Can you work these out from the model? Positions are in its coordinate system, mm. Face numbers are marked on the shaded views. A direction names the side the tool comes from. Give positions to 0.01 mm unless a question says otherwise; leave off trailing zeros. Loops run counter-clockwise (first coordinate to the right, second up) from the corner with the lowest first, then second, coordinate; pieces in that order, holes last. Notation, with made-up numbers: (43.5, 49.25) - (62.5, 49.25) arc R15 ccw to (62.5, 61.25) - close; hole circle Ø11 at (14.25, -0.75). An arc over 180 degrees is marked (long way). Answer as a JSON object with one key per item and string values.
```python
from build123d import *

# Parameters (mm, degrees)
SKETCH1_W                   = 114.3
SKETCH1_H                   = 127
BOSS_EXTRUDE1_DEPTH         = 6.35
SKETCH2_W                   = 9.398
SKETCH2_H                   = 101.6
BOSS_EXTRUDE2_DEPTH         = 29.21
SKETCH10_R                  = 3.175
CUT_EXTRUDE1_DEPTH          = 115.596583549
SKETCH13_W                  = 2.667
SKETCH13_H                  = 6.35
CUT_EXTRUDE2_DEPTH          = 9.398
CUT_EXTRUDE3_REACH          = 92.286
SKETCH15_W                  = 25.4
SKETCH15_H                  = 25.4
MIRROR4_COPY_1_SKETCH_W     = 2.667
MIRROR4_COPY_1_SKETCH_H     = 6.35
MIRROR4_COPY_1_DEPTH        = 9.398
SKETCH19_W                  = 1.524
SKETCH19_H                  = 43.18
CUT_EXTRUDE4_DEPTH          = 5.08
SKETCH23_W                  = 5.842
SKETCH23_H                  = 11.43
CUT_EXTRUDE5_DEPTH          = 20.828
SKETCH24_W                  = 127.881325932
SKETCH24_H                  = 16.190143287
CUT_EXTRUDE6_DEPTH          = 12.7
SKETCH26_W                  = 20.33012471
SKETCH26_H                  = 111.91731712
CUT_EXTRUDE8_DEPTH          = 25.781
CHAMFER1_SIZE               = 3.81
SKETCH28_W                  = 17.78
SKETCH28_H                  = 12.7
BOSS_EXTRUDE3_DEPTH         = 12.7
SKETCH30_W                  = 11.43
SKETCH30_H                  = 5.842
CUT_EXTRUDE9_DEPTH          = 75.423408732
F_1_4_CLEARANCE_HOLE1_D     = 7.14248
F_1_4_CLEARANCE_HOLE1_DEPTH = 3.636839777
CHAMFER3_SIZE2              = 6.35
CHAMFER3_SIZE               = 2.54
F_1_4_CLEARANCE_HOLE2_D     = 7.14248
F_1_4_CLEARANCE_HOLE2_DEPTH = 15.24


with BuildPart() as part:
    # Sketch1 → Boss-Extrude1 (new body)
    with BuildSketch(Plane.XY):
        Rectangle(SKETCH1_W, SKETCH1_H)
    extrude(amount=BOSS_EXTRUDE1_DEPTH)

    # Sketch2 → Boss-Extrude2 (add)
    with BuildSketch(Plane.XY.offset(6.35)):
        with Locations((26.67, 0)):
            Rectangle(SKETCH2_W, SKETCH2_H)
    boss_extrude2 = extrude(amount=BOSS_EXTRUDE2_DEPTH)

    # Mirror1: Boss-Extrude2 across plane
    add(boss_extrude2.mirror(Plane(origin=(0, 0, 0), x_dir=(0, 0, 1), z_dir=(1, 0, 0))))

    # Sketch10 → Cut-Extrude1 (cut, through all)
    with BuildSketch(Plane(origin=(31.369, 0, 0), x_dir=(0, 0, -1), z_dir=(1, 0, 0))):
        with Locations((-22.86, 43.18)):
            Circle(SKETCH10_R)
    cut_extrude1 = extrude(amount=-CUT_EXTRUDE1_DEPTH, mode=Mode.SUBTRACT)

    # Mirror2: Cut-Extrude1 across plane
    add(cut_extrude1.mirror(Plane.ZX), mode=Mode.SUBTRACT)

    # Sketch13 → Cut-Extrude2 (cut)
    with BuildSketch(Plane(origin=(31.369, 0, 0), x_dir=(0, 0, -1), z_dir=(1, 0, 0))):
        with Locations((-30.5435, 43.18)):
            Rectangle(SKETCH13_W, SKETCH13_H)
    cut_extrude2 = extrude(amount=-CUT_EXTRUDE2_DEPTH, mode=Mode.SUBTRACT)

    # Sketch15 → Cut-Extrude3 (cut, up to next)
    with BuildSketch(Plane.XY.offset(6.35), mode=Mode.PRIVATE) as cut_extrude3_sk1:
        with Locations((-5.08, 0)):
            Rectangle(SKETCH15_W, SKETCH15_H)
    cut_extrude3_tool1 = extrude(cut_extrude3_sk1.sketch, amount=-CUT_EXTRUDE3_REACH, mode=Mode.PRIVATE) & part.part
    add(cut_extrude3_tool1.solids().sort_by_distance((-5.08, 0, 6.35))[0], mode=Mode.SUBTRACT)

    # Sketch16 → #4 Clearance Hole1 (revolve, cut)
    with BuildSketch(Plane(origin=(26.67, 43.18, 35.56), x_dir=(0, -1, 0), z_dir=(1, 0, 0))):
        Polygon((0, 0), (0, 12.918574487), (1.63195, 11.938), (1.63195, 0), align=None)
    f_4_clearance_hole1 = revolve(axis=Axis((26.67, 43.18, 41.91), (0, 0, -1)), mode=Mode.SUBTRACT)

    # Mirror3: Cut-Extrude2, #4 Clearance Hole1 across plane
    add(cut_extrude2.mirror(Plane(origin=(0, 0, 0), x_dir=(0, 0, 1), z_dir=(1, 0, 0))), mode=Mode.SUBTRACT)
    add(f_4_clearance_hole1.mirror(Plane(origin=(0, 0, 0), x_dir=(0, 0, 1), z_dir=(1, 0, 0))), mode=Mode.SUBTRACT)

    # Mirror4: Cut-Extrude2, #4 Clearance Hole1 across plane
    add(cut_extrude2.mirror(Plane.ZX), mode=Mode.SUBTRACT)
    add(f_4_clearance_hole1.mirror(Plane.ZX), mode=Mode.SUBTRACT)

    # Mirror4 copy 1 sketch → Mirror4 copy 1 (cut)
    with BuildSketch(Plane(origin=(-31.369, 0, 0), x_dir=(0, 0, -1), z_dir=(-1, 0, 0))):
        with Locations((-30.5435, 43.18)):
            Rectangle(MIRROR4_COPY_1_SKETCH_W, MIRROR4_COPY_1_SKETCH_H)
    extrude(amount=-MIRROR4_COPY_1_DEPTH, mode=Mode.SUBTRACT)

    # Mirror4 copy 2 sketch → Mirror4 copy 2 (revolve, cut)
    with BuildSketch(Plane(origin=(-26.67, -43.18, 35.56), x_dir=(0, 1, 0), z_dir=(-1, 0, 0))):
        Polygon((0, 0), (0, 12.918574487), (1.63195, 11.938), (1.63195, 0), align=None)
    revolve(axis=Axis((-26.67, -43.18, 41.91), (0, 0, -1)), mode=Mode.SUBTRACT)

    # Sketch19 → Cut-Extrude4 (cut)
    with BuildSketch(Plane(origin=(-21.971, 0, 0), x_dir=(0, 0, -1), z_dir=(1, 0, 0))):
        with Locations((-22.86, 0)):
            Rectangle(SKETCH19_W, SKETCH19_H)
    extrude(amount=-CUT_EXTRUDE4_DEPTH, mode=Mode.SUBTRACT)

    # Sketch23 → Cut-Extrude5 (cut)
    with BuildSketch(Plane.XY.offset(35.56)):
        with Locations((26.67, 0)):
            Rectangle(SKETCH23_W, SKETCH23_H)
    extrude(amount=-CUT_EXTRUDE5_DEPTH, mode=Mode.SUBTRACT)

    # Sketch24 → Cut-Extrude6 (cut)
    with BuildSketch(Plane(origin=(0, 63.5, 0), x_dir=(1, 0, 0), z_dir=(0, 1, 0))):
        with Locations((0, -3.427395894)):
            Rectangle(SKETCH24_W, SKETCH24_H)
    cut_extrude6 = extrude(amount=-CUT_EXTRUDE6_DEPTH, mode=Mode.SUBTRACT)

    # Mirror5: Cut-Extrude6 across plane
    add(cut_extrude6.mirror(Plane.ZX), mode=Mode.SUBTRACT)

    # Sketch26 → Cut-Extrude8 (cut)
    with BuildSketch(Plane(origin=(57.15, 0, 0), x_dir=(0, 0, -1), z_dir=(1, 0, 0))):
        with Locations((-3.366450344, 0)):
            Rectangle(SKETCH26_W, SKETCH26_H)
    cut_extrude8 = extrude(amount=-CUT_EXTRUDE8_DEPTH, mode=Mode.SUBTRACT)

    # Mirror6: Cut-Extrude8 across plane
    add(cut_extrude8.mirror(Plane(origin=(0, 0, 0), x_dir=(0, 0, 1), z_dir=(1, 0, 0))), mode=Mode.SUBTRACT)

    # Chamfer1
    chamfer1_edges = [part.edges().sort_by_distance(p)[0] for p in [
        (0, 50.8, 0),
    ]]
    chamfer(chamfer1_edges, length=CHAMFER1_SIZE)

    # Sketch28 → Boss-Extrude3 (add)
    with BuildSketch(Plane.XZ.offset(50.8)):
        with Locations((0, 6.35)):
            Rectangle(SKETCH28_W, SKETCH28_H)
    extrude(amount=BOSS_EXTRUDE3_DEPTH)

    # Sketch30 → Cut-Extrude9 (cut, through all)
    with BuildSketch(Plane.XY.offset(12.7)):
        with Locations((0.067049503, -56.942160223)):
            Rectangle(SKETCH30_W, SKETCH30_H)
    extrude(amount=-CUT_EXTRUDE9_DEPTH, mode=Mode.SUBTRACT)

    # 1/4 Clearance Hole1
    with Locations(Plane(origin=(0, -63.5, 0), x_dir=(-1, 0, 0), z_dir=(0, -1, 0))):
        with Locations((0, -6.35)):
            Hole(F_1_4_CLEARANCE_HOLE1_D / 2, depth=F_1_4_CLEARANCE_HOLE1_DEPTH)

    # Chamfer3
    chamfer3_edges = [part.edges().sort_by_distance(p)[0] for p in [
        (0, -50.8, 12.7),
    ]]
    chamfer3_side = [part.faces().sort_by_distance(p)[0] for p in [
        (0, -50.8508, 12.7),
    ]]
    chamfer(chamfer3_edges, length=CHAMFER3_SIZE - 0.0001, length2=CHAMFER3_SIZE2 - 0.0001, reference=chamfer3_side[0])  # a hair under: the kernel refuses the full size

    # 1/4 Clearance Hole2
    with Locations(Plane(origin=(31.369, 0, 0), x_dir=(0, 0, -1), z_dir=(1, 0, 0))):
        with Locations((-21.082, 0)):
            Hole(F_1_4_CLEARANCE_HOLE2_D / 2, depth=F_1_4_CLEARANCE_HOLE2_DEPTH)


solid = part.part
```
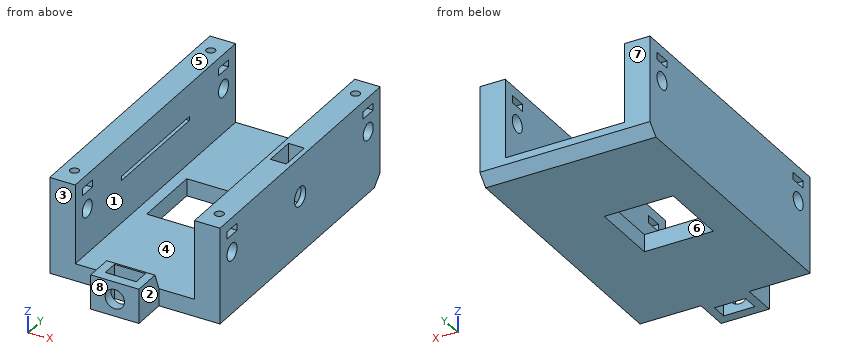
1) I'm going to push flat-ended pins straight in: P1, Ø1.3, axis at x = 28.5, z = 30.5, coming from the -Y side; P2, Ø12, axis at x = 2.5, y = 26.5, coming from the +Z side; P3, Ø14, axis at y = -59, z = 6, coming from the -X side. Where does each tip first touch, or does it pass through?
Check sheet entries:
{"P1": "y = -50.8", "P2": "z = 6.35", "P3": "x = -8.89"}
2) I need wall thicknesses on L1, parallel to X at y = 43, z = 34; L2, parallel to Y at x = -26.67, z = 27.45; L3, parallel to X at y = -36, z = 27.5. Which ranges of each line are inside material? Lowest first, please.
Check sheet entries:
{"L1": "-31.37 to -28.29, -25.05 to -21.97, 21.97 to 25.05, 28.29 to 31.37", "L2": "-50.8 to -44.81, -41.55 to 41.55, 44.81 to 50.8", "L3": "-31.37 to -21.97, 21.97 to 31.37"}
3) Imagine slicing it at C-C on y = -26.5. Write out the boundary of the cut face in (x, z).
Check sheet entries:
{"outline": "(-31.37, 0) - (31.37, 0) - (31.37, 35.56) - (21.97, 35.56) - (21.97, 6.35) - (-21.97, 6.35) - (-21.97, 35.56) - (-31.37, 35.56) - close"}
4) Imagine slicing it at A-A on x = -15. Write out the boundary of the cut face in (y, z), and give its area (3 significant figures).
Check sheet entries:
{"outline": "(-50.8, 0) - (-12.7, 0) - (-12.7, 6.35) - (-50.8, 6.35) - close; (12.7, 0) - (46.99, 0) - (50.8, 3.81) - (50.8, 6.35) - (12.7, 6.35) - close", "area": "477 mm2"}
5) Which directions (+Z, -Z, +X, -X, +Y, -Y) give clear straight access to the entire face, cutting with the end or side of a thin tool? Please do the marked faces 1, 2, 3 and 4.
Check sheet entries:
{"face 1": "+Z, +Y, -Y", "face 2": "+Z, -Z, +X, -Y", "face 3": "+Z, -Z, -X, -Y", "face 4": "+Z, +Y"}
6) Imagine slicing it at D-D on y = 2. Write out the boundary of the cut face in (x, z), and give its area (3 significant figures).
Check sheet entries:
{"outline": "(-31.37, 0) - (-17.78, 0) - (-17.78, 6.35) - (-21.97, 6.35) - (-21.97, 22.1) - (-27.05, 22.1) - (-27.05, 23.62) - (-21.97, 23.62) - (-21.97, 35.56) - (-31.37, 35.56) - close; (7.62, 0) - (31.37, 0) - (31.37, 18.12) - (29.59, 18.12) - (29.59, 14.73) - (23.75, 14.73) - (23.75, 18.12) - (21.97, 18.12) - (21.97, 6.35) - (7.62, 6.35) - close; (21.97, 24.04) - (23.75, 24.04) - (23.75, 35.56) - (21.97, 35.56) - close; (29.59, 24.04) - (31.37, 24.04) - (31.37, 35.56) - (29.59, 35.56) - close", "area": "636 mm2"}
7) If we mould it in two halves opening along Y, with no side actions, what happens to the marked faces 5, 6, 7 and 8? For each: released by +Y, released by -Y, zero draft, split by the parting line, or undercut.
Check sheet entries:
{"face 5": "zero draft", "face 6": "undercut", "face 7": "released by +Y", "face 8": "released by -Y"}
